from build123d import *

# Parameters (mm, degrees)
SKETCH1_W           = 150
SKETCH1_H           = 300
SKETCH1_R           = 10
BOSS_EXTRUDE1_DEPTH = 10


with BuildPart() as part:
    # Sketch1 → Boss-Extrude1 (new body)
    with BuildSketch(Plane.XY):
        Rectangle(SKETCH1_W, SKETCH1_H)
        with Locations((0, -107)):
            Circle(SKETCH1_R, mode=Mode.SUBTRACT)
    extrude(amount=BOSS_EXTRUDE1_DEPTH)


solid = part.part
Check sheet for the modelled part. Datum: model origin and axes. Units: mm. Give positions to 0.01 mm unless a question says otherwise; leave off trailing zeros. Write each loop counter-clockwise with the first axis right and the second up, starting at its lowest first coordinate (ties: lowest second). Pieces come first, ordered by that corner, then holes. Notation, with made-up numbers: (-7.75, 66.25) -> (13.25, 66.25) arc R19 cw to (13.25, 90.25) -> close; hole circle Ø2 at (44.25, 6). An arc over 180 degrees is marked (long way). Write item = value, one per line.
Item 1: Sectioned sample at B-B on y = -107. Record the boundary of the cut face in (x, z), and give its area (3 significant figures).
Output:
outline = (-75, 0) -> (-10, 0) -> (-10, 10) -> (-75, 10) -> close; (10, 0) -> (75, 0) -> (75, 10) -> (10, 10) -> close
area = 1,300 mm^2
Item 2: Release check for a two-part mould opening along X. For faces 1 (the flat face through (-1, 2, 10)), 2 (the cylindrical face through (-1.302, -97.085, 4.93)), 3 (the flat face through (75, -2, 5)), 4 (the flat face through (-75, -2, 5)) record: +X half, -X half, draft (parallel to the pull), parting line (faces both ways), or undercut.
Output:
face_1 = draft
face_2 = undercut
face_3 = +X half
face_4 = -X half
Item 3: Scan lines: probe 1 along Y at (x, z) = (0, 7.5); probe 2 along X at (y, z) = (-110.5, 2.5); probe 3 along Y at (x, z) = (-6.5, 1.5). Record each from-to range of solid material in increasing order. Write a range as from..to.
Output:
probe_1 = -150..-117, -97..150
probe_2 = -75..-9.37, 9.37..75
probe_3 = -150..-114.6, -99.4..150
Item 4: Sectioned sample at A-A on x = 0. Record the boundary of the cut face in (y, z), and give its area (3 significant figures).
Output:
outline = (-150, 0) -> (-117, 0) -> (-117, 10) -> (-150, 10) -> close; (-97, 0) -> (150, 0) -> (150, 10) -> (-97, 10) -> close
area = 2,800 mm^2
